Verification items for the finished model (mm, model axes). Give positions to 0.01 mm unless a question says otherwise; leave off trailing zeros. Loops run counter-clockwise (first coordinate to the right, second up) from the corner with the lowest first, then second, coordinate; pieces in that order, holes last. Notation, with made-up numbers: M 7.25,-33 L 23.25,-33 A25 cw 23.25,1 Z; hole C 74,-37.5 d4. An arc over 180 degrees is marked long. Write each question's results on one line, items separated by ' | '. Start each with the question number.
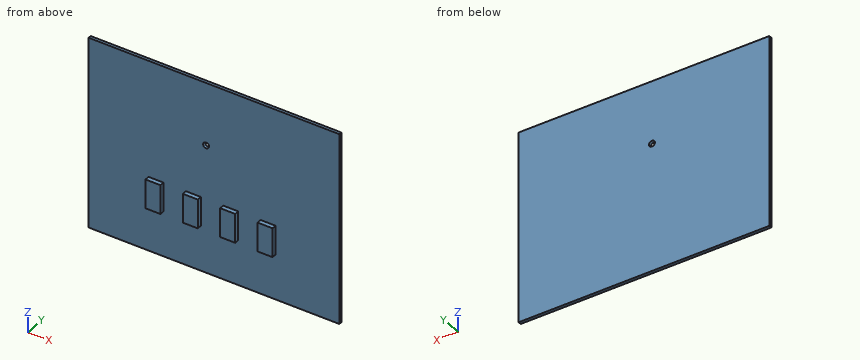
```python
from build123d import *

# Parameters (mm, degrees)
SKETCH_3_W          = 167.68
SKETCH_3_H          = 130
EXTRUDE_1_DEPTH     = 2
SKETCH_5_R          = 2
CUT_EXTRUDE_1_DEPTH = 2
SKETCH_6_W          = 10
SKETCH_6_H          = 19.7733087
EXTRUDE_2_DEPTH     = 3


with BuildPart() as part:
    # 스케치3 → 보스-돌출1 (new body)
    with BuildSketch(Plane.XZ.offset(15)):
        with Locations((38.84, -35)):
            Rectangle(SKETCH_3_W, SKETCH_3_H)
    extrude(amount=EXTRUDE_1_DEPTH)

    # 스케치5 → 컷-돌출1 (cut)
    with BuildSketch(Plane.XZ.offset(17)):
        with Locations((33.535545215, -12.778353339)):
            Circle(SKETCH_5_R)
    extrude(amount=-CUT_EXTRUDE_1_DEPTH, mode=Mode.SUBTRACT)

    # 스케치6 → 보스-돌출2 (add)
    with BuildSketch(Plane.XZ.offset(17)):
        with Locations((0, -59.389009604)):
            Rectangle(SKETCH_6_W, SKETCH_6_H)
        with Locations((25, -59.389009604)):
            Rectangle(SKETCH_6_W, SKETCH_6_H)
        with Locations((50, -59.389009604)):
            Rectangle(SKETCH_6_W, SKETCH_6_H)
        with Locations((75, -59.389009604)):
            Rectangle(SKETCH_6_W, SKETCH_6_H)
    extrude(amount=EXTRUDE_2_DEPTH)


solid = part.part
```
1. Section check A-A, the plane y = -17.9. Record the boundary of the cut face in (x, z).
2. Thickness scan on probe 1 along X at (y, z) = (-19.25, -69); probe 2 along Z at (x, y) = (74, -18.4); probe 3 along Y at (x, z) = (114, -63). Record the ranges inside material, lowest first.
3. Section check D-D, the plane z = -42.5. Record the boundary of the cut face in (x, y).
4. Section check C-C, the plane z = -59.5. Record the boundary of the cut face in (x, y).
5. Depth check by flat-ended pin: pin 1 Ø2.5 at (y, z) = (-19, -58) entering from -X; pin 2 Ø2.5 at (y, z) = (-19, -62.5) entering from +X; pin 3 Ø1.5 at (x, y) = (0.5, -19) entering from -Z. Enter the tip coordinate at first touch or a pass-through.
6. Section check B-B, the plane x = 51.5. Record the boundary of the cut face in (y, z), plus the area to 3 significant figures.
Filled sheet:
1) outline: M -5,-69.28 L 5,-69.28 L 5,-49.5 L -5,-49.5 Z; M 20,-69.28 L 30,-69.28 L 30,-49.5 L 20,-49.5 Z; M 45,-69.28 L 55,-69.28 L 55,-49.5 L 45,-49.5 Z; M 70,-69.28 L 80,-69.28 L 80,-49.5 L 70,-49.5 Z
2) probe 1: -5 to 5, 20 to 30, 45 to 55, 70 to 80 | probe 2: -69.28 to -49.5 | probe 3: -17 to -15
3) outline: M -45,-17 L 122.68,-17 L 122.68,-15 L -45,-15 Z
4) outline: M -45,-17 L -5,-17 L -5,-20 L 5,-20 L 5,-17 L 20,-17 L 20,-20 L 30,-20 L 30,-17 L 45,-17 L 45,-20 L 55,-20 L 55,-17 L 70,-17 L 70,-20 L 80,-20 L 80,-17 L 122.68,-17 L 122.68,-15 L -45,-15 Z
5) pin 1: x = -5 | pin 2: x = 80 | pin 3: z = -69.28
6) outline: M -20,-69.28 L -17,-69.28 L -17,-100 L -15,-100 L -15,30 L -17,30 L -17,-49.5 L -20,-49.5 Z | area: 319 mm2
